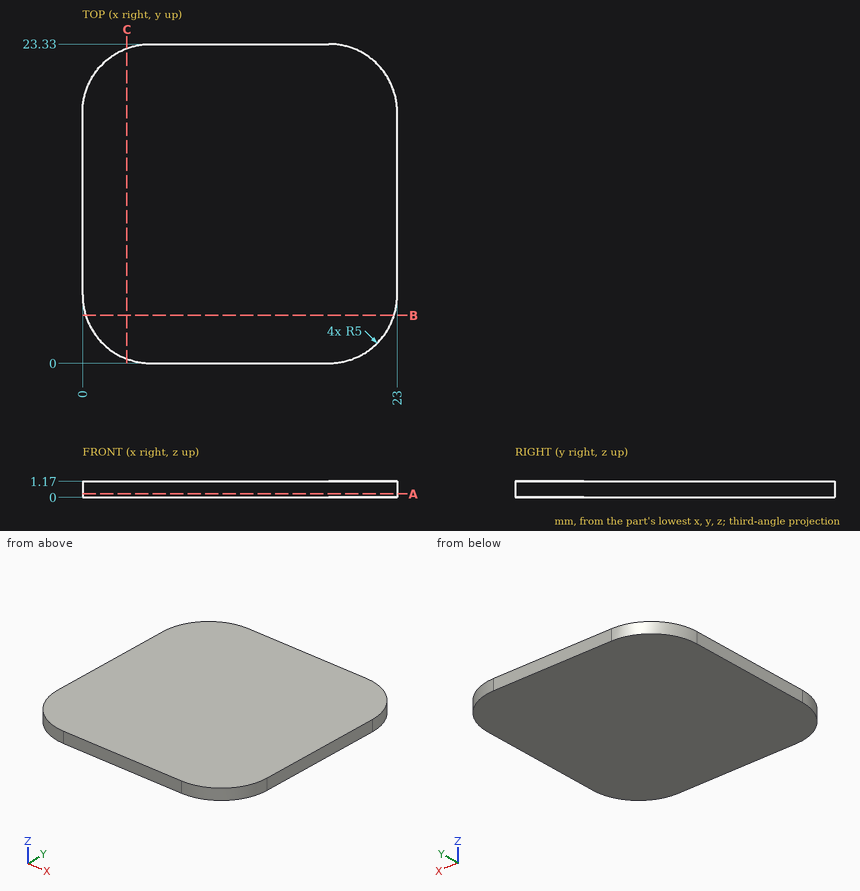
Can you work these out from the drawing? Everything is in mm from the part's minimum corner. Give positions to 0.01 mm unless a question says otherwise; leave off trailing zeros. Loops run counter-clockwise (first coordinate to the right, second up) from the corner with the lowest first, then second, coordinate; pieces in that order, holes last. Notation, with made-up numbers: M 15.5,86 L 46.5,86 A4 ccw 46.5,90 Z; hole C 69.5,27.25 d4. An arc over 180 degrees is marked long. Use CSV: the item, a comma, the result in double quotes. Start each with the question number.
1. If I drill on L1, parallel to X at y = 20.5, z = 0.45; L2, parallel to Y at x = 20.25, z = 0.4; L3, parallel to Y at x = 1.5, z = 0.85, over which ranges is the centre line in solid material (lowest first)?
2. Imagine slicing it at B-B, the plane y = 3.5. Write out the boundary of the cut face in (x, z), plus the area to 3 significant figures.
3. Imagine slicing it at A-A, the plane z = 0.25. Write out the boundary of the cut face in (x, y).
4. Imagine slicing it at C-C, the plane x = 3.25. Write out the boundary of the cut face in (y, z).
Response values:
1,L1,"0.5 to 22.5"
1,L2,"0.53 to 22.8"
1,L3,"1.43 to 21.9"
2,outline,"M 0.23,0 L 22.77,0 L 22.77,1.17 L 0.23,1.17 Z"
2,area,"26.4 mm^2"
3,outline,"M 0,5 A5 ccw 5,0 L 18,0 A5 ccw 23,5 L 23,18.33 A5 ccw 18,23.33 L 5,23.33 A5 ccw 0,18.33 Z"
4,outline,"M 0.32,0 L 23.01,0 L 23.01,1.17 L 0.32,1.17 Z"
